Verification items for the finished model (mm, model axes). Give positions to 0.01 mm unless a question says otherwise; leave off trailing zeros. Loops run counter-clockwise (first coordinate to the right, second up) from the corner with the lowest first, then second, coordinate; pieces in that order, holes last. Notation, with made-up numbers: M 35.25,19 L 50.25,19 A15 cw 50.25,28 Z; hole C 4.5,84 d3. An arc over 180 degrees is marked long. Use CSV: the item, a comma, the result in double quotes.
from build123d import *

# Parameters (mm, degrees)
DODANIE_WYCI_GNI_CIE1_DEPTH = 2
SZKIC2_W                    = 5
SZKIC2_H                    = 16
WYTNIJ_WYCI_GNI_CIE1_DEPTH  = 5
WYTNIJ_WYCI_GNI_CIE2_DEPTH  = 10
WYTNIJ_WYCI_GNI_CIE3_DEPTH  = 10


with BuildPart() as part:
    # Szkic1 → Dodanie-wyciągnięcie1 (new body)
    with BuildSketch(Plane.XY):
        Polygon((39.660703644, 7.348041155), (39.998203889, -8.651958845), (67.367690874, -8.651958845), (67.367690874, 7.348041155), align=None)
    extrude(amount=-DODANIE_WYCI_GNI_CIE1_DEPTH)

    # Szkic2 → Wytnij-wyciągnięcie1 (cut)
    with BuildSketch(Plane.XY):
        with Locations((64.867690874, -0.651958845)):
            Rectangle(SZKIC2_W, SZKIC2_H)
    extrude(amount=-WYTNIJ_WYCI_GNI_CIE1_DEPTH, mode=Mode.SUBTRACT)

    # Szkic3 → Wytnij-wyciągnięcie2 (cut)
    with BuildSketch(Plane.XY):
        with BuildLine():
            Line((39.660703644, 7.348041155), (39.998203889, -8.651958845))
            Line((39.998203889, -8.651958845), (48.125210145, -8.651958845))
            ThreePointArc((48.125210145, -8.651958845), (51.694710699, -0.869414217), (49.289973229, 7.348041155))
            Line((49.289973229, 7.348041155), (39.660703644, 7.348041155))
        make_face()
    extrude(amount=-WYTNIJ_WYCI_GNI_CIE2_DEPTH, mode=Mode.SUBTRACT)

    # Szkic4 → Wytnij-wyciągnięcie3 (cut)
    with BuildSketch(Plane.XY):
        with BuildLine():
            Line((48.125210145, -8.651958845), (51.027201312, -8.651958845))
            ThreePointArc((51.027201312, -8.651958845), (54.184885403, -0.707437008), (51.322077756, 7.348041155))
            Line((51.322077756, 7.348041155), (49.289973229, 7.348041155))
            Line((49.289973229, 7.348041155), (48.125210145, -8.651958845))
        make_face()
    extrude(amount=-WYTNIJ_WYCI_GNI_CIE3_DEPTH, mode=Mode.SUBTRACT)


solid = part.part
(1) Section check B-B on z = -0.9. Record the cut outline in (x, y), plus the area to 3 significant figures.
Calculated:
outline,"M 51.03,-8.65 L 62.37,-8.65 L 62.37,7.35 L 51.32,7.35 A12.14 cw Z"
area,"146 mm²"
(2) Mould release check, pull along Y, two halves, no side actions. Record for faces 1 (the flat face through (62.368, -1, -1)), 2 (the flat face through (57, -8.652, -1)), 3 (the flat face through (57, 7.348, -1)), 4 (the cylindrical face through (54.182, -0.83, -0.986)): released by +Y, released by -Y, zero draft, split by the parting line, or undercut.
Calculated:
face 1,"zero draft"
face 2,"released by -Y"
face 3,"released by +Y"
face 4,"undercut"
(3) Section check C-C on x = 51.75. Record the cut outline in (y, z), plus the area to 3 significant figures.
Calculated:
outline,"M -8.65,-2 L -7.78,-2 L -7.78,0 L -8.65,0 Z; M 6.81,-2 L 7.35,-2 L 7.35,0 L 6.81,0 Z"
area,"2.82 mm²"
(4) Section check D-D on y = 6.75. Record the cut outline in (x, z), plus the area to 3 significant figures.
Calculated:
outline,"M 51.8,-2 L 62.37,-2 L 62.37,0 L 51.8,0 Z"
area,"21.1 mm²"
(5) Scan lines: L1, parallel to Y at x = 52.25, z = -1.3; L2, parallel to Y at x = 51.75, z = -0.95; L3, parallel to X at y = -0.5, z = -0.95. Record each from-to range of solid material in increasing order. Write a range as from..to.
Calculated:
L1,"y = -8.65..-7.06, 6.09..7.35"
L2,"y = -8.65..-7.78, 6.81..7.35"
L3,"x = 54.19..62.37"
(6) Section check A-A on x = 53. Record the cut outline in (y, z).
Calculated:
outline,"M -8.65,-2 L -5.72,-2 L -5.72,0 L -8.65,0 Z; M 4.75,-2 L 7.35,-2 L 7.35,0 L 4.75,0 Z"
